Here's how the part is built. I have some questions about the finished solid (model axes, mm). A direction names the side the tool comes from. Coordinates: 2 decimals unless noted, no trailing zeros. Loops run counter-clockwise (first coordinate to the right, second up) from the corner with the lowest first, then second, coordinate; pieces in that order, holes last. Notation, with made-up numbers: M 71.25,56 L 90.25,56 A26 ccw 90.25,86 Z; hole C 38.5,49 d4. An arc over 180 degrees is marked long. Use CSV: the item, a comma, the result in double quotes. Start each with the question number.
Q1. If we section it at C-C (y = 1): State how many separate pieces and enclosed holes the cut face has, and give its area (3 significant figures).
Q2. Please list where these lines run through material, in increasing order: probe 1 along Z at (x, y) = (17, 4); probe 2 along Z at (x, y) = (-2, 0.5); probe 3 along X at (y, z) = (3.5, -117.5). Write a range as [from, to].
Q3. If we section it at B-B (z = -78): Please give me the cut outline in (x, y).
Q4. For pin 1 Ø3 at (x, y) = (-17.5, 5.5) entering from -Z; pin 2 Ø3 at (y, z) = (2, -77) entering from +X, each with a flat end and sliding along its axis, tell me the tip position at first contact or that it passes through.
Q5. Which directions (+Z, -Z, +X, -X, +Y, -Y) give clear straight access to the entire face, cutting with the end or side of a thin tool? Please do faces 1 (the flat face through (-19, 3, -76)), 2 (the flat face through (-31.29, 3.13, -100.73)).
Q6. If we section it at A-A (x = 8.5): Please give me the cut outline in (y, z).
Q7. If we mould it in two halves opening along Z, with no side actions, what happens to faces 3 (the flat face through (0, 6.35, -106)), 4 (the cylindrical face through (0.92, 3.22, -220.98)), 5 (the flat face through (31.185, 3.131, -97.951))? For each: +Z half, -Z half, draft (parallel to the pull), parting line (faces both ways), or undercut.
from build123d import *

# Parameters (mm, degrees)
BOSS_EXTRUDE1_DEPTH     = 6.35
SKETCH2_R               = 2.6
CUT_EXTRUDE1_DEPTH      = 238.676928834
ESQUISSE3_R             = 21
ENL_V_MAT_EXTRU_2_DEPTH = 238.676928834
ESQUISSE7_R             = 1.5
ENL_V_MAT_EXTRU_3_DEPTH = 238.676928834
CUT_EXTRUDE3_DEPTH      = 238.676928834
SKETCH5_R               = 2
CUT_EXTRUDE4_DEPTH      = 238.676928834


with BuildPart() as part:
    # Sketch1 → Boss-Extrude1 (new body)
    with BuildSketch(Plane(origin=(0, 0, 0), x_dir=(1, 0, 0), z_dir=(0, 1, 0))):
        with BuildLine():
            Line((27.5, 0), (34.975254116, 198.684097441))
            ThreePointArc((34.975254116, 198.684097441), (0, 235), (-34.975254116, 198.684097441))
            Line((-34.975254116, 198.684097441), (-27.5, 0))
            ThreePointArc((-27.5, 0), (0, -27.5), (27.5, 0))
        make_face()
    extrude(amount=BOSS_EXTRUDE1_DEPTH)

    # Sketch2 → Cut-Extrude1 (cut, through all)
    with BuildSketch(Plane(origin=(0, 6.35, 0), x_dir=(1, 0, 0), z_dir=(0, 1, 0))):
        with Locations(Location((0, 0, 0), (0, 0, 270))):
            Circle(SKETCH2_R)
    extrude(amount=-CUT_EXTRUDE1_DEPTH, mode=Mode.SUBTRACT)

    # Esquisse3 → Enlèv. mat.-Extru.2 (cut, through all)
    with BuildSketch(Plane(origin=(0, 6.35, 0), x_dir=(1, 0, 0), z_dir=(0, 1, 0))):
        with Locations(Location((0, 200, 0), (0, 0, 270))):
            Circle(ESQUISSE3_R)
    extrude(amount=-ENL_V_MAT_EXTRU_2_DEPTH, mode=Mode.SUBTRACT)

    # Esquisse7 → Enlèv. mat.-Extru.3 (cut, through all)
    with BuildSketch(Plane(origin=(0, 6.35, 0), x_dir=(1, 0, 0), z_dir=(0, 1, 0))):
        with Locations(Location((-19.339370465, 219.339370465, 0), (0, 0, 270))):
            Circle(ESQUISSE7_R)
        with Locations(Location((19.339370465, 219.339370465, 0), (0, 0, 270))):
            Circle(ESQUISSE7_R)
        with Locations(Location((19.339370465, 180.660629535, 0), (0, 0, 270))):
            Circle(ESQUISSE7_R)
        with Locations(Location((-19.339370465, 180.660629535, 0), (0, 0, 270))):
            Circle(ESQUISSE7_R)
    extrude(amount=-ENL_V_MAT_EXTRU_3_DEPTH, mode=Mode.SUBTRACT)

    # Sketch4 → Cut-Extrude3 (cut, through all)
    with BuildSketch(Plane(origin=(0, 6.35, 0), x_dir=(1, 0, 0), z_dir=(0, 1, 0))):
        with BuildLine():
            Line((-19, 56.7), (-19, 96.7))
            ThreePointArc((-19, 96.7), (-15, 100.7), (-11, 96.7))
            Line((-11, 96.7), (-11, 56.7))
            ThreePointArc((-11, 56.7), (-15, 52.7), (-19, 56.7))
        make_face()
    extrude(amount=-CUT_EXTRUDE3_DEPTH, mode=Mode.SUBTRACT)

    # Sketch5 → Cut-Extrude4 (cut, through all)
    with BuildSketch(Plane.XZ):
        with Locations(Location((15.5, -117.5, 0), (0, 0, 270))):
            Circle(SKETCH5_R)
        with Locations(Location((15.5, -148.5, 0), (0, 0, 270))):
            Circle(SKETCH5_R)
        with Locations(Location((-15.5, -148.5, 0), (0, 0, 270))):
            Circle(SKETCH5_R)
        with Locations(Location((-15.5, -117.5, 0), (0, 0, 270))):
            Circle(SKETCH5_R)
    extrude(amount=-CUT_EXTRUDE4_DEPTH, mode=Mode.SUBTRACT)


solid = part.part
Results below:
1,separate pieces,"1"
1,enclosed holes,"11"
1,area,"13,800 mm^2"
2,probe 1,"[-230.59, -212.33], [-187.67, -149.82], [-147.18, -118.82], [-116.18, 21.62]"
2,probe 2,"[-234.94, -220.9], [-179.1, -1.66], [1.66, 27.43]"
2,probe 3,"[-31.92, -17.5], [-13.5, 13.5], [17.5, 31.92]"
3,outline,"M -30.43,0 L -19,0 L -19,6.35 L -30.43,6.35 Z; M -11,0 L 30.43,0 L 30.43,6.35 L -11,6.35 Z"
4,pin 1,"z = -231.13"
4,pin 2,"x = 30.45"
5,face 1,"+Y, -Y"
5,face 2,"+Z, -X, +Y, -Y"
6,outline,"M 0,-233.95 L 6.35,-233.95 L 6.35,-219.2 L 0,-219.2 Z; M 0,-180.8 L 6.35,-180.8 L 6.35,26.15 L 0,26.15 Z"
7,face 3,"draft"
7,face 4,"undercut"
7,face 5,"+Z half"
